Source: CAD feature listing. Evaluate the final solid. Frame: model axes, mm. Coordinates: 2 decimals unless noted, no trailing zeros. Loops run counter-clockwise (first coordinate to the right, second up) from the corner with the lowest first, then second, coordinate; pieces in that order, holes last.
Item 1: Section query B-B, the plane y = 25.4. Return the cut outline in (x, z).
Item 2: Section query C-C, the plane z = 431.8. Return the cut outline in (x, y).
Item 3: Pin query (flat end, axial travel): pin 1 Ø14.5 at (y, z) = (31.5, 117.5) entering from +X. Return the tip coordinate at first contact, or that it passes through.
Item 4: Line query: probe 1 along Y at (x, z) = (10.25, 119); probe 2 along Z at (x, y) = (6.35, 50.5); probe 3 along X at (y, z) = (35, 335). Output: solid intervals per line, ascending.
Item 5: Section query D-D, the plane z = 184. Return the cut outline in (x, y), then the cut area to 3 significant figures.
Item 6: Section query A-A, the plane x = 6.35. Return the cut outline in (y, z), then the cut area to 3 significant figures.
Autodesk Inventor part; units mm, degrees
ref_plane "YZ Plane" through (0, 0, 0) normal (1, 0, 0) x (0, 1, 0)
ref_plane "XZ Plane" through (0, 0, 0) normal (0, 1, 0) x (-1, 0, 0)
ref_plane "XY Plane" through (0, 0, 0) normal (0, 0, 1) x (1, 0, 0)
sketch "Sketch1" plane through (0, 0, 0) normal (0, 0, 1) x (1, 0, 0)
  line L0 (0, 0) -> (12.7, 0)
  line L1 (12.7, 50.8) -> (0, 50.8)
  line L2 (0, 50.8) -> (0, 0)
  line L3 (12.7, 1.27) -> (1.27, 1.27)
  line L4 (1.27, 1.27) -> (1.27, 49.53)
  line L5 (1.27, 49.53) -> (12.7, 49.53)
  line L6 (12.7, 0) -> (12.7, 1.27)
  line L7 (12.7, 49.53) -> (12.7, 50.8)
  dimension "d0" = 12.7
  dimension "d1" = 50.8
  dimension "d2" = 11.43
  dimension "d3" = 48.26
extrude "Extrusion1" add sketch "Sketch1" along normal blind 457.2
sketch "Sketch2" plane through (0, 0, 0) normal (-1, 0, 0) x (0, 0, 1)
  circle A0 centre (25.4, 25.4) radius 14.2875
  circle A1 centre (431.8, 25.4) radius 14.2875
  point P0 (0, 0)
  dimension "d6" = 28.575
  dimension "d7" = 28.575
extrude "Extrusion2" cut sketch "Sketch2" against normal through all
sketch "Sketch3" plane through (0, 50.8, 0) normal (0, 1, 0) x (1, 0, 0)
  line L0 (12.7237, -456.4581) -> (12.7, -253.2581)
  line L1 (12.7, 0) -> (12.7, -457.2)
  line L2 (0, 0) -> (0, -457.2)
  circle A0 centre (6.35, -253.2581) radius 3.0861
  dimension "d12" = 6.1722
extrude "Extrusion3" cut sketch "Sketch3" against normal blind 12.7
equation "\"d4\" = u1"
equation "\"u1\" = 457.2"
properties part number "VerseFrameCChannel 18in"
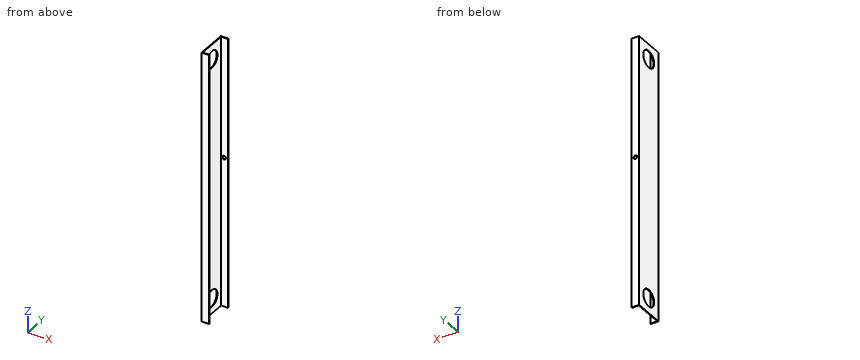
Verdict:
1. outline: (0, 0) - (1.27, 0) - (1.27, 11.11) - (0, 11.11) - close; (0, 39.69) - (1.27, 39.69) - (1.27, 417.51) - (0, 417.51) - close; (0, 446.09) - (1.27, 446.09) - (1.27, 457.2) - (0, 457.2) - close
2. outline: (0, 0) - (12.7, 0) - (12.7, 1.27) - (1.27, 1.27) - (1.27, 11.11) - (0, 11.11) - close; (0, 39.69) - (1.27, 39.69) - (1.27, 49.53) - (12.7, 49.53) - (12.7, 50.8) - (0, 50.8) - close
3. pin 1: stops at x = 1.27
4. probe 1: y = 0 to 1.27, 49.53 to 50.8
4. probe 2: z = 0 to 250.17, 256.34 to 457.2
4. probe 3: x = 0 to 1.27
5. outline: (0, 0) - (12.7, 0) - (12.7, 1.27) - (1.27, 1.27) - (1.27, 49.53) - (12.7, 49.53) - (12.7, 50.8) - (0, 50.8) - close
5. area: 93.5 mm2
6. outline: (0, 0) - (1.27, 0) - (1.27, 457.2) - (0, 457.2) - close; (49.53, 0) - (50.8, 0) - (50.8, 250.17) - (49.53, 250.17) - close; (49.53, 256.34) - (50.8, 256.34) - (50.8, 457.2) - (49.53, 457.2) - close
6. area: 1,150 mm2
